from build123d import *

# Parameters (mm, degrees)
SKETCH1_W           = 26.67
SKETCH1_H           = 52.07
BOSS_EXTRUDE1_DEPTH = 6.35
FILLET1_R           = 6.35


with BuildPart() as part:
    # Sketch1 → Boss-Extrude1 (new body)
    with BuildSketch(Plane.XY):
        with BuildLine():
            Line((12.7, -63.5), (0, -63.5))
            Line((0, -63.5), (0, -120.671250195))
            Line((0, -120.671250195), (12.7, -120.671250195))
            Line((12.7, -120.671250195), (12.7, -112.971250195))
            ThreePointArc((12.7, -112.971250195), (7.7, -107.971250195), (12.7, -102.971250195))
            Line((12.7, -102.971250195), (12.7, -87.571250195))
            ThreePointArc((12.7, -87.571250195), (7.7, -82.571250195), (12.7, -77.571250195))
            Line((12.7, -77.571250195), (12.7, -63.5))
        make_face()
        with BuildLine():
            Line((25.4, -63.5), (12.7, -63.5))
            Line((12.7, -63.5), (12.7, -77.571250195))
            ThreePointArc((12.7, -77.571250195), (16.235533906, -79.035716289), (17.7, -82.571250195))
            ThreePointArc((17.7, -82.571250195), (16.235533906, -86.106784101), (12.7, -87.571250195))
            Line((12.7, -87.571250195), (12.7, -102.971250195))
            ThreePointArc((12.7, -102.971250195), (16.235533906, -104.435716289), (17.7, -107.971250195))
            ThreePointArc((17.7, -107.971250195), (16.235533906, -111.506784101), (12.7, -112.971250195))
            Line((12.7, -112.971250195), (12.7, -120.671250195))
            Line((12.7, -120.671250195), (25.4, -120.671250195))
            Line((25.4, -120.671250195), (25.4, -100.271250195))
            ThreePointArc((25.4, -100.271250195), (20.4, -95.271250195), (25.4, -90.271250195))
            Line((25.4, -90.271250195), (25.4, -63.5))
        make_face()
        with BuildLine():
            Line((38.1, -120.671250195), (38.1, -63.5))
            Line((38.1, -63.5), (25.4, -63.5))
            Line((25.4, -63.5), (25.4, -90.271250195))
            ThreePointArc((25.4, -90.271250195), (28.935533906, -91.735716289), (30.4, -95.271250195))
            ThreePointArc((30.4, -95.271250195), (28.935533906, -98.806784101), (25.4, -100.271250195))
            Line((25.4, -100.271250195), (25.4, -120.671250195))
            Line((25.4, -120.671250195), (38.1, -120.671250195))
        make_face()
        Polygon((38.1, 0), (0, 0), (0, -63.5), (12.7, -63.5), (25.4, -63.5), (38.1, -63.5), align=None)
        with Locations((19.05, -31.75)):
            Rectangle(SKETCH1_W, SKETCH1_H, mode=Mode.SUBTRACT)
    extrude(amount=BOSS_EXTRUDE1_DEPTH)

    # Fillet1
    fillet1_edges = [part.edges().sort_by_distance(p)[0] for p in [
        (0, -120.671250195, 3.175),
        (0, 0, 3.175),
        (38.1, 0, 3.175),
        (38.1, -120.671250195, 3.175),
    ]]
    fillet(fillet1_edges, radius=FILLET1_R)


solid = part.part
Part model, mm, in its own coordinate system. A direction names the side the tool comes from. Give positions to 0.01 mm unless a question says otherwise; leave off trailing zeros. Order: outer loops, then holes, each group sorted by start corner. A loop starts at its lowest first (then second) coordinate and runs counter-clockwise, first axis right, second up. Notation, with made-up numbers: (-10, -9) - (1, -9) arc R17 cw to (1, 6) - close; hole circle Ø10 at (12, -25.75). An arc over 180 degrees is marked (long way). Use a Markdown table: item, result.
1) Flat gauge pins, fed straight in: P1, Ø2, axis at x = 23.5, y = -58, coming from the -Z side; P2, Ø8, axis at x = 13.5, y = -48.5, coming from the +Z side. Where does each tip first touch, or does it go through?
Checked values:
| item | result |
|---|---|
| P1 | z = 0 |
| P2 | through |
2) Saw through at A-A on y = -43.5. List the corners of the cut face in (x, z) (3 decimals), plus the area to 3 significant figures.
Checked values:
| item | result |
|---|---|
| outline | (0, 0) - (5.715, 0) - (5.715, 6.35) - (0, 6.35) - close; (32.385, 0) - (38.1, 0) - (38.1, 6.35) - (32.385, 6.35) - close |
| area | 72.6 mm² |
3) 3-axis set-ups, long thin cutter, end or side, ignore diameter. For faces 5 (the flat face through (38.1, -61, 3)), 6 (the flat face through (19, -5.715, 3)): which of +Z, -Z, +X, -X, +Y, -Y reach the whole face in a straight line?
Checked values:
| item | result |
|---|---|
| face 5 | +Z, -Z, +X, +Y, -Y |
| face 6 | +Z, -Z |
4) Saw through at B-B on z = 3. List the corners of the cut face in (x, y) (3 decimals).
Checked values:
| item | result |
|---|---|
| outline | (0, -114.321) arc R6.35 ccw to (6.35, -120.671) - (31.75, -120.671) arc R6.35 ccw to (38.1, -114.321) - (38.1, -6.35) arc R6.35 ccw to (31.75, 0) - (6.35, 0) arc R6.35 ccw to (0, -6.35) - close; hole (5.715, -57.785) - (32.385, -57.785) - (32.385, -5.715) - (5.715, -5.715) - close; hole circle Ø10 at (12.7, -107.971); hole circle Ø10 at (12.7, -82.571); hole circle Ø10 at (25.4, -95.271) |
5) Two-plate mould, pull along X, no slides. Class faces 1 (the flat face through (32.385, -32, 3)), 2 (the cylindrical face through (1.91, -118.86, 3.22)), 3 (the flat face through (5.715, -32, 3)), 4 (the flat face through (19, 0, 3)): +X half, -X half, draft (parallel to the pull), parting line (faces both ways), or undercut.
Checked values:
| item | result |
|---|---|
| face 1 | undercut |
| face 2 | -X half |
| face 3 | undercut |
| face 4 | draft |
6) Saw through at C-C on x = 10. List the corners of the cut face in (y, z) (3 decimals), plus the area to 3 significant figures.
Checked values:
| item | result |
|---|---|
| outline | (-120.671, 0) - (-112.18, 0) - (-112.18, 6.35) - (-120.671, 6.35) - close; (-103.763, 0) - (-86.78, 0) - (-86.78, 6.35) - (-103.763, 6.35) - close; (-78.363, 0) - (-57.785, 0) - (-57.785, 6.35) - (-78.363, 6.35) - close; (-5.715, 0) - (0, 0) - (0, 6.35) - (-5.715, 6.35) - close |
| area | 329 mm² |
7) Saw through at D-D on x = 27. List the corners of the cut face in (y, z) (3 decimals), plus the area to 3 significant figures.
Checked values:
| item | result |
|---|---|
| outline | (-120.671, 0) - (-100.008, 0) - (-100.008, 6.35) - (-120.671, 6.35) - close; (-90.534, 0) - (-57.785, 0) - (-57.785, 6.35) - (-90.534, 6.35) - close; (-5.715, 0) - (0, 0) - (0, 6.35) - (-5.715, 6.35) - close |
| area | 375 mm² |
8) Probe L1, parallel to Y at x = 13, z = 3 (3 decimals); L2, parallel to X at y = -15, z = 2.5 (3 decimals); L3, parallel to Y at x = 24.5, z = 2.5 (3 decimals). List the from-to ranges inside material, lowest first. Write a range as from..to.
Checked values:
| item | result |
|---|---|
| L1 | -120.671..-112.962, -102.98..-87.562, -77.58..-57.785, -5.715..0 |
| L2 | 0..5.715, 32.385..38.1 |
| L3 | -120.671..-100.19, -90.353..-57.785, -5.715..0 |
